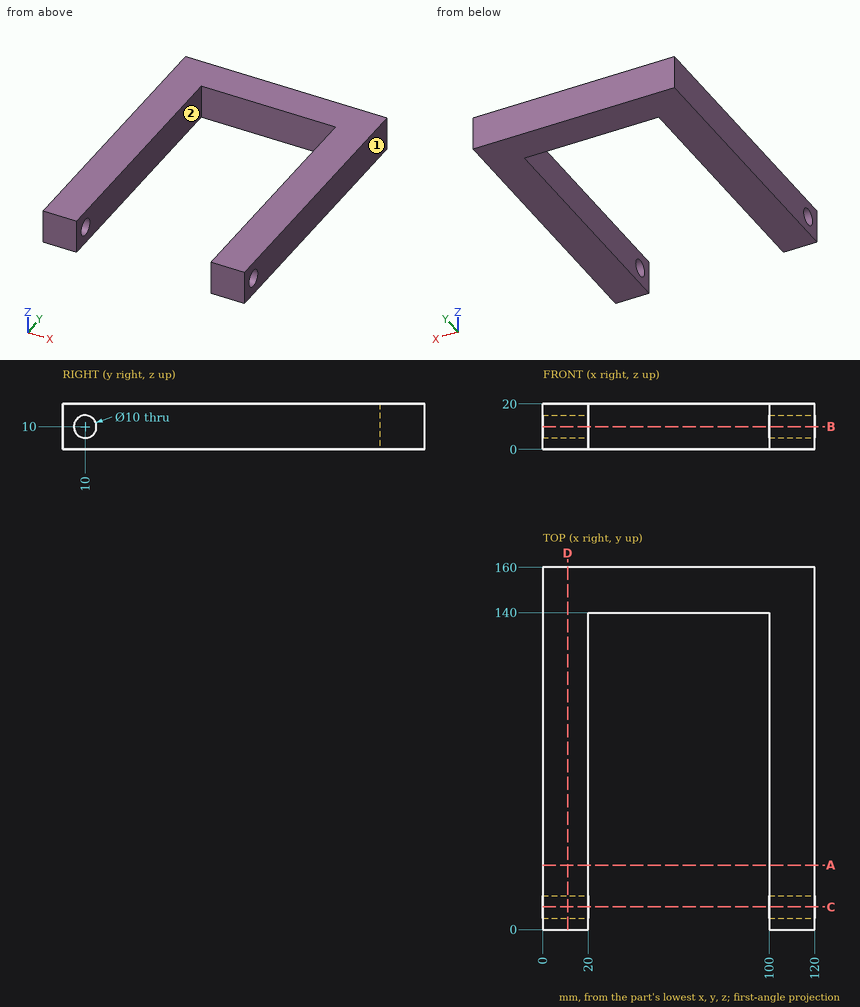
Input: dimensioned drawing with shaded views. Units: mm. Origin: part minimum x, y, z. A direction names the side the tool comes from. Give positions to 0.01 mm unless a question says otherwise; leave off trailing zeros. Write each loop counter-clockwise with the first axis right and the second up, starting at its lowest first coordinate (ties: lowest second). Pieces come first, ordered by that corner, then holes.
1. Material intervals for line 1 along X through (y, z) = (123, 17.5); line 2 along Z through (x, y) = (6.75, 10); line 3 along Y through (x, z) = (25.5, 14), sorted ascending.
2. Section query B-B (z = 10). Return the cut outline in (x, y).
3. Section query A-A (y = 28.5). Return the cut outline in (x, z), then the cut area to 3 significant figures.
4. First-contact query: pin 1 (8 mm diameter, centred on x = 95, z = 16.5, fed in from -Y). Flat tip, straight axial feed; report the tip coordinate or a pass-through.
5. Section query D-D (x = 11). Return the cut outline in (y, z).
6. Section query C-C (y = 10). Return the cut outline in (x, z), then the cut area to 3 significant figures.
7. Access query for the marked faces 1 and 2. Directions: +Z, -Z, +X, -X, +Y, -Y. A direction counts if a zero-diameter tool reaches every point of the face in a straight line with its end or side. Return the directions, or none.
Output values:
1. line 1: x = 0 to 20, 100 to 120
1. line 2: z = 0 to 5, 15 to 20
1. line 3: y = 140 to 160
2. outline: (0, 0) - (20, 0) - (20, 5) - (0, 5) - close; (0, 15) - (20, 15) - (20, 140) - (100, 140) - (100, 15) - (120, 15) - (120, 160) - (0, 160) - close; (100, 0) - (120, 0) - (120, 5) - (100, 5) - close
3. outline: (0, 0) - (20, 0) - (20, 20) - (0, 20) - close; (100, 0) - (120, 0) - (120, 20) - (100, 20) - close
3. area: 800 mm2
4. pin 1: stops at y = 140
5. outline: (0, 0) - (160, 0) - (160, 20) - (0, 20) - close; hole circle Ø10 at (10, 10)
6. outline: (0, 0) - (20, 0) - (20, 5) - (0, 5) - close; (0, 15) - (20, 15) - (20, 20) - (0, 20) - close; (100, 0) - (120, 0) - (120, 5) - (100, 5) - close; (100, 15) - (120, 15) - (120, 20) - (100, 20) - close
6. area: 400 mm2
7. face 1: +Z, -Z, +X, +Y, -Y
7. face 2: +Z, -Z, -Y
